Here's the drawing with two shaded views (mm, measured from the low corner). I have some questions. Round coordinates to 2 decimals unless told otherwise and drop trailing zeros. Loops run counter-clockwise (first coordinate to the right, second up) from the corner with the lowest first, then second, coordinate; pieces in that order, holes last. Notation, with made-up numbers: M -39.75,12.5 L -5.75,12.5 A33 cw -5.75,44.5 Z; hole C 64,61.25 d4. An arc over 180 degrees is marked long. One line per item, written item: value. Start each with the question number.
Q1. Please list where these lines run through material, in increasing order: line 1 along X through (y, z) = (172.5, 1.55); line 2 along Y through (x, z) = (11, 1); line 3 along Y through (x, z) = (208, 1.85).
Q2. Imagine slicing it at B-B (y = 80). Please give me the cut outline in (x, z), then the cut area to 3 significant figures.
Q3. Imagine slicing it at C-C (z = 0.95). Please give me the cut outline in (x, y).
Q4. Imagine slicing it at A-A (x = 82). Please give me the cut outline in (y, z), then the cut area to 3 significant figures.
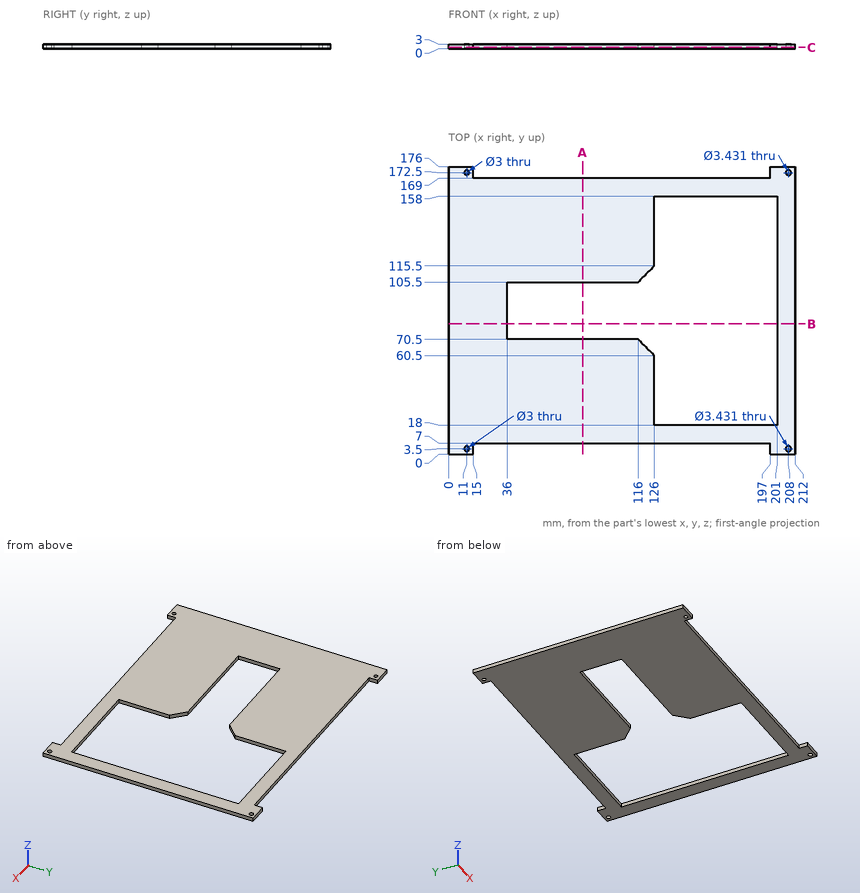
Report:
1. line 1: x = 0 to 9.5, 12.5 to 15, 197 to 206.28, 209.72 to 212
1. line 2: y = 0 to 2, 5 to 171, 174 to 176
1. line 3: y = 0 to 1.78, 5.22 to 170.78, 174.22 to 176
2. outline: M 0,0 L 36,0 L 36,3 L 0,3 Z; M 201,0 L 212,0 L 212,3 L 201,3 Z
2. area: 141 mm²
3. outline: M 0,0 L 15,0 L 15,7 L 197,7 L 197,0 L 212,0 L 212,176 L 197,176 L 197,169 L 15,169 L 15,176 L 0,176 Z; hole C 11,3.5 d3; hole C 11,172.5 d3; hole M 36,70.5 L 116,70.5 L 126,60.5 L 126,18 L 201,18 L 201,158 L 126,158 L 126,115.5 L 116,105.5 L 36,105.5 Z; hole C 208,3.5 d3.43; hole C 208,172.5 d3.43
4. outline: M 7,0 L 70.5,0 L 70.5,3 L 7,3 Z; M 105.5,0 L 169,0 L 169,3 L 105.5,3 Z
4. area: 381 mm²
